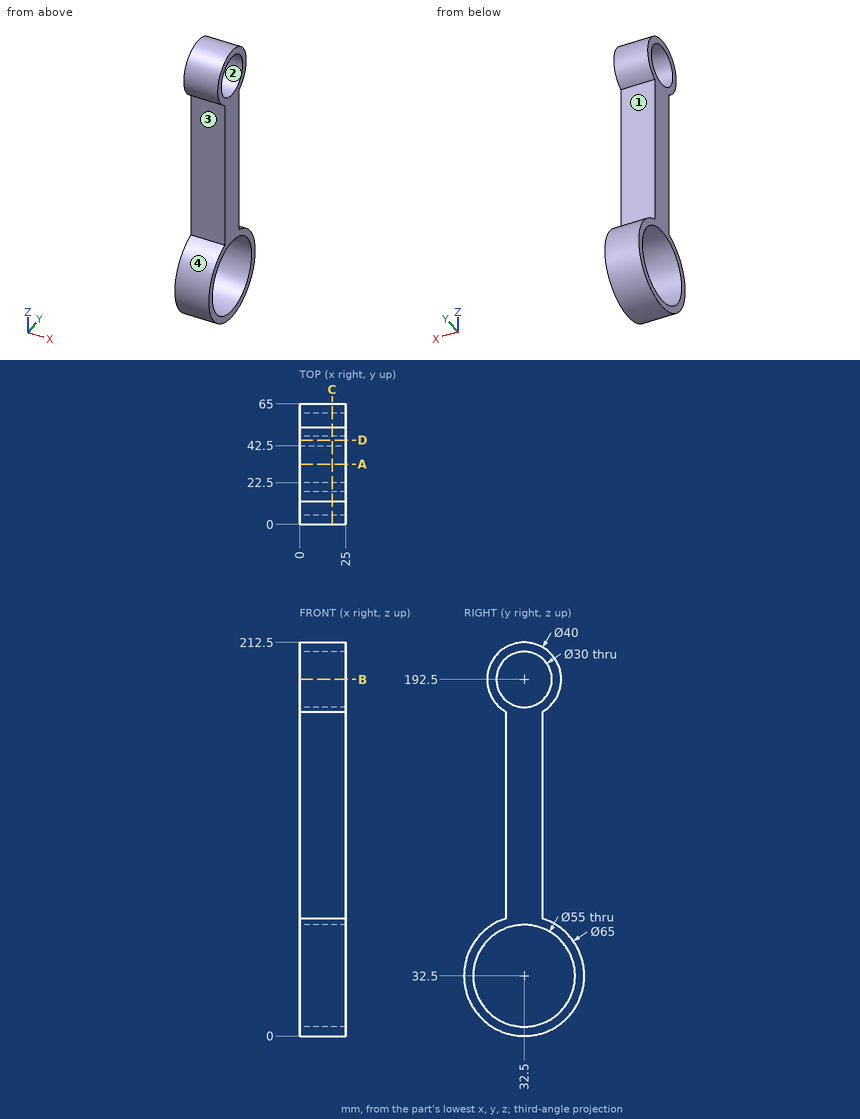
Verification items for this drawing (mm, ordinates from the low corner). A direction names the side the tool comes from. Coordinates: 2 decimals unless noted, no trailing zeros. Loops run counter-clockwise (first coordinate to the right, second up) from the corner with the lowest first, then second, coordinate; pieces in that order, holes last. Notation, with made-up numbers: (-38, -19.75) - (-18, -19.75) arc R17 cw to (-18, 2.25) - close; hole circle Ø4 at (-7.5, -22.5). An arc over 180 degrees is marked (long way). One line per item, written item: value. Start each with the question number.
(1) Cross-section at D-D on y = 45.5. Enter the section's corners in (x, z), plus the area to 3 significant figures.
(2) Cross-section at A-A on y = 32.5. Enter the section's corners in (x, z).
(3) Cross-section at C-C on x = 17.5. Enter the section's corners in (y, z), plus the area to 3 significant figures.
(4) Cross-section at B-B on z = 192.5. Enter the section's corners in (x, y).
(5) Depth check by flat-ended pin: P1, Ø1, axis at x = 13, z = 125.5, coming from the +Y side; P2, Ø3, axis at x = 6, z = 190.5, coming from the -Y side; P3, Ø4, axis at y = 50, z = 60, coming from the -X side; P4, Ø1, axis at x = 8.5, y = 13.5, coming from the +Z side. Enter the tip coordinate at first touch or a pass-through.
(6) Tool access check on the marked faces 3 and 4. Record the directions out of +Z, -Z, +X, -X, +Y, -Y that give a thin tool (end or side, any length) a straight path to the whole face; none if there is none.
(7) Material ranges on line 1 (Z direction, x = 15, y = 32.5); line 2 (Z direction, x = 12.25, y = 22); line 3 (Y direction, x = 19, z = 32), recorded low to high. Write a range as [from, to].
(8) Mould release check, pull along Z, two halves, no side actions. Record for the marked faces 1 and 2: released by +Z, released by -Z, zero draft, split by the parting line, or undercut.
Results below:
1. outline: (0, 2.71) - (25, 2.71) - (25, 8.27) - (0, 8.27) - close; (0, 56.73) - (25, 56.73) - (25, 62.29) - (0, 62.29) - close; (0, 177.3) - (25, 177.3) - (25, 185.02) - (0, 185.02) - close; (0, 199.98) - (25, 199.98) - (25, 207.7) - (0, 207.7) - close
1. area: 663 mm2
2. outline: (0, 0) - (25, 0) - (25, 5) - (0, 5) - close; (0, 60) - (25, 60) - (25, 177.5) - (0, 177.5) - close; (0, 207.5) - (25, 207.5) - (25, 212.5) - (0, 212.5) - close
3. outline: (22.5, 63.42) arc R32.5 ccw (long way) to (42.5, 63.42) - (42.5, 175.18) arc R20 ccw (long way) to (22.5, 175.18) - close; hole circle Ø55 at (32.5, 32.5); hole circle Ø30 at (32.5, 192.5)
3. area: 3,670 mm2
4. outline: (0, 12.5) - (25, 12.5) - (25, 17.5) - (0, 17.5) - close; (0, 47.5) - (25, 47.5) - (25, 52.5) - (0, 52.5) - close
5. P1: stops at y = 42.5
5. P2: stops at y = 12.51
5. P3: stops at x = 0
5. P4: stops at z = 200.1
6. face 3: +X, -X, -Y
6. face 4: +X, -X
7. line 1: z = [0, 5], [60, 177.5], [207.5, 212.5]
7. line 2: z = [1.74, 7.08], [57.92, 63.26], [175.48, 181.79], [203.21, 209.52]
7. line 3: y = [0, 5], [60, 65]
8. face 1: undercut
8. face 2: undercut
